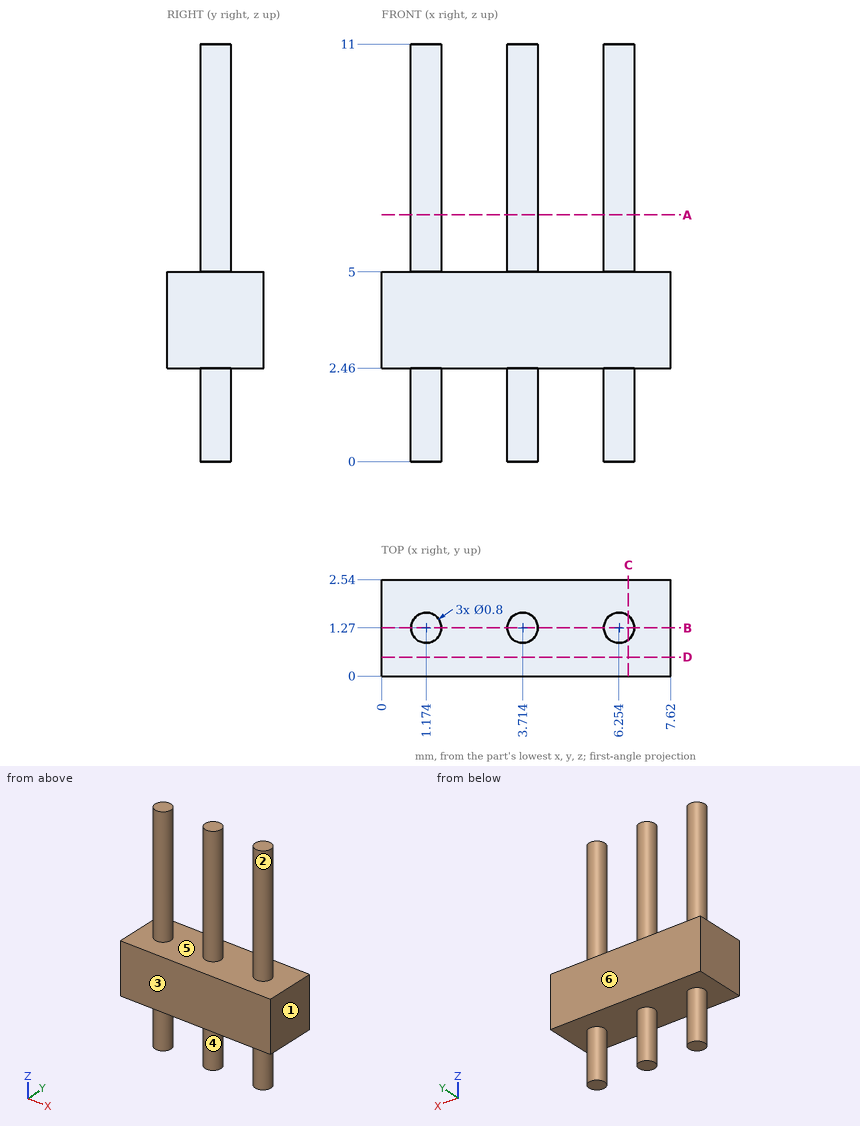
Drawing for the job (mm, zero at the part's lowest x, y, z). A direction names the side the tool comes from. Give positions to 0.01 mm unless a question says otherwise; leave off trailing zeros. Loops run counter-clockwise (first coordinate to the right, second up) from the corner with the lowest first, then second, coordinate; pieces in that order, holes last.
(1) Band-saw the part on C-C (x = 6.5). Write the cut outline in (y, z) (1 decimal).
Return value:
outline: (0, 2.5) - (1, 2.5) - (1, 0) - (1.6, 0) - (1.6, 2.5) - (2.5, 2.5) - (2.5, 5) - (1.6, 5) - (1.6, 11) - (1, 11) - (1, 5) - (0, 5) - close
(2) Band-saw the part on D-D (y = 0.5). Write the cut outline in (x, z).
Return value:
outline: (0, 2.46) - (7.62, 2.46) - (7.62, 5) - (0, 5) - close
(3) Band-saw the part on B-B (y = 1.27). Write the cut outline in (x, z) (1 decimal).
Return value:
outline: (0, 2.5) - (0.8, 2.5) - (0.8, 0) - (1.6, 0) - (1.6, 2.5) - (3.3, 2.5) - (3.3, 0) - (4.1, 0) - (4.1, 2.5) - (5.9, 2.5) - (5.9, 0) - (6.7, 0) - (6.7, 2.5) - (7.6, 2.5) - (7.6, 5) - (6.7, 5) - (6.7, 11) - (5.9, 11) - (5.9, 5) - (4.1, 5) - (4.1, 11) - (3.3, 11) - (3.3, 5) - (1.6, 5) - (1.6, 11) - (0.8, 11) - (0.8, 5) - (0, 5) - close
(4) 3-axis set-ups, long thin cutter, end or side, ignore diameter. For the marked faces 4, 5 and 6: which of +Z, -Z, +X, -X, +Y, -Y reach the whole face in a straight line?
Return value:
face 4: -Z
face 5: +Z
face 6: +Z, -Z, +X, -X, +Y
(5) Pin check, flat tips, straight feed: pin 1 (1.5 mm diameter, centred on y = 1, z = 6.5, fed in from +X); pin 2 (1.3 mm diameter, centred on x = 2, y = 1, fed in from -Z); pin 3 (1.5 mm diameter, centred on x = 4.5, z = 7, fed in from -Y). Stop position of each tip, or through.
Return value:
pin 1: stops at x = 6.65
pin 2: stops at z = 0
pin 3: stops at y = 0.87
(6) Band-saw the part on A-A (z = 6.5). Write the cut outline in (x, y) (1 decimal).
Return value:
outline: circle Ø0.8 at (1.2, 1.3); circle Ø0.8 at (3.7, 1.3); circle Ø0.8 at (6.3, 1.3)
(7) Pull direction X, two halves, no side cores. Call the marked faces 1, 2 and 3: pulls with the +X half, pulls with the -X half, needs draft (parallel to the pull), parting line crosses it, or undercut.
Return value:
face 1: pulls with the +X half
face 2: undercut
face 3: needs draft
(8) Drill centre lines: line 1 along X through (y, z) = (1.3, 1) (1 decimal); line 2 along Z through (x, y) = (0.5, 0.5); line 3 along Y through (x, z) = (4, 9). Where is each one in solid material? Low to high.
Return value:
line 1: x = 0.8 to 1.6, 3.3 to 4.1, 5.9 to 6.7
line 2: z = 2.46 to 5
line 3: y = 0.99 to 1.55
